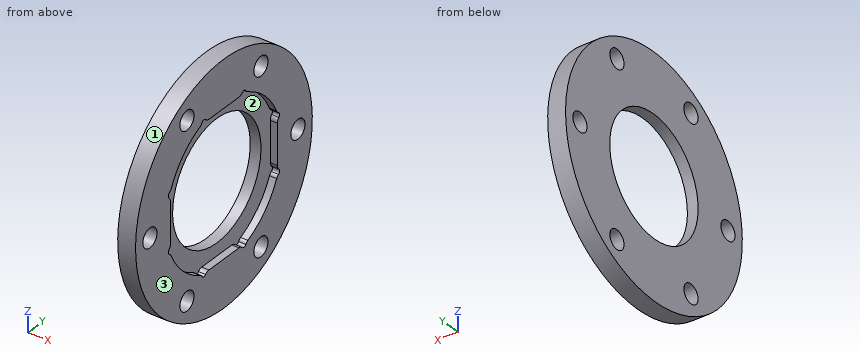
```python
from build123d import *

# Parameters (mm, degrees)
SKETCH_3_R          = 20
EXTRUDE_3_DEPTH     = 3
SKETCH_4_R          = 13.1
CUT_EXTRUDE_1_DEPTH = 1.2
EXTRUDE_START       = 1.2
EXTRUDE_4_DEPTH     = 1.2
SKETCH_6_R          = 10
CUT_EXTRUDE_2_DEPTH = 29.341489022
SKETCH_7_R          = 1.6
CUT_EXTRUDE_4_DEPTH = 29.442925307
SKETCH_8_R          = 0.5
CUT_EXTRUDE_5_DEPTH = 1.2
FILLET_START        = 1.8
FILLET_1_DEPTH      = 2.2


with BuildPart() as part:
    # 草图3 → 凸台-拉伸3 (new body)
    with BuildSketch(Plane(origin=(0, 0, 0), x_dir=(0, 0, -1), z_dir=(1, 0, 0))):
        Circle(SKETCH_3_R)
    extrude(amount=EXTRUDE_3_DEPTH)

    # 草图4 → 切除-拉伸1 (cut)
    with BuildSketch(Plane(origin=(3, 0, 0), x_dir=(0, 0, -1), z_dir=(1, 0, 0))):
        Circle(SKETCH_4_R)
    extrude(amount=-CUT_EXTRUDE_1_DEPTH, mode=Mode.SUBTRACT)

    # 草图5 → 凸台-拉伸4 (add)
    with BuildSketch(Plane(origin=(1.8, 0, 0), x_dir=(0, 0, -1), z_dir=(1, 0, 0)).offset(EXTRUDE_START)):
        with BuildLine():
            Line((-5.019960159, 12.1), (5.019960159, 12.1))
            ThreePointArc((5.019960159, 12.1), (0, 13.1), (-5.019960159, 12.1))
        make_face()
        with BuildLine():
            Line((-12.1, 5.019960159), (-12.1, -5.019960159))
            ThreePointArc((-12.1, -5.019960159), (-13.1, 0), (-12.1, 5.019960159))
        make_face()
        with BuildLine():
            Line((-5.019960159, -12.1), (5.019960159, -12.1))
            ThreePointArc((5.019960159, -12.1), (0, -13.1), (-5.019960159, -12.1))
        make_face()
        with BuildLine():
            Line((12.1, 5.019960159), (12.1, -5.019960159))
            ThreePointArc((12.1, -5.019960159), (13.1, 0), (12.1, 5.019960159))
        make_face()
    extrude(amount=-EXTRUDE_4_DEPTH)

    # 草图6 → 切除-拉伸2 (cut, through all)
    with BuildSketch(Plane(origin=(1.8, 0, 0), x_dir=(0, 0, -1), z_dir=(1, 0, 0))):
        Circle(SKETCH_6_R)
    extrude(amount=-CUT_EXTRUDE_2_DEPTH, mode=Mode.SUBTRACT)

    # 草图7 → 切除-拉伸4 (cut, through all)
    with BuildSketch(Plane(origin=(3, 0, 0), x_dir=(0, 0, -1), z_dir=(1, 0, 0))):
        with Locations((0, 16.75)):
            Circle(SKETCH_7_R)
        with Locations((14.505925513, 8.375)):
            Circle(SKETCH_7_R)
        with Locations((14.505925513, -8.375)):
            Circle(SKETCH_7_R)
        with Locations((0, -16.75)):
            Circle(SKETCH_7_R)
        with Locations((-14.505925513, -8.375)):
            Circle(SKETCH_7_R)
        with Locations((-14.505925513, 8.375)):
            Circle(SKETCH_7_R)
    extrude(amount=-CUT_EXTRUDE_4_DEPTH, mode=Mode.SUBTRACT)

    # 草图8 → 切除-拉伸5 (cut)
    with BuildSketch(Plane(origin=(3, 0, 0), x_dir=(0, 0, -1), z_dir=(1, 0, 0))):
        with Locations((-4.519960159, 12.1)):
            Circle(SKETCH_8_R)
        with Locations((12.1, 4.519960159)):
            Circle(SKETCH_8_R)
        with Locations((4.519960159, -12.1)):
            Circle(SKETCH_8_R)
        with Locations((-12.1, -4.519960159)):
            Circle(SKETCH_8_R)
        with Locations((4.519960159, 12.1)):
            Circle(SKETCH_8_R)
        with Locations((12.1, -4.519960159)):
            Circle(SKETCH_8_R)
        with Locations((-4.519960159, -12.1)):
            Circle(SKETCH_8_R)
        with Locations((-12.1, 4.519960159)):
            Circle(SKETCH_8_R)
    extrude(amount=-CUT_EXTRUDE_5_DEPTH, mode=Mode.SUBTRACT)

    # 圆角1: read off the stored shape, not the designer's step
    # 圆角1 outline → 圆角1 (cut)
    with BuildSketch(Plane.YZ.offset(FILLET_START)):
        with BuildLine():
            ThreePointArc((3.40192617, -12.1), (3.810174461, -12.187129071), (4.147282163, -12.433333333))
            ThreePointArc((4.147282163, -12.433333333), (4.05287398, -12.278411045), (4.019960159, -12.1))
            Line((4.019960159, -12.1), (3.40192617, -12.1))
        make_face()
        with BuildLine():
            ThreePointArc((5.019960159, -12.1), (5.003372821, -12.227719215), (4.954711368, -12.346964343))
            ThreePointArc((4.954711368, -12.346964343), (5.149921864, -12.102428131), (5.411148977, -11.930191396))
            ThreePointArc((5.411148977, -11.930191396), (5.216245603, -12.016687639), (5.019960159, -12.1))
        make_face()
        with BuildLine():
            ThreePointArc((-4.147282163, -12.433333333), (-3.810174461, -12.187129071), (-3.40192617, -12.1))
            Line((-3.40192617, -12.1), (-4.019960159, -12.1))
            ThreePointArc((-4.019960159, -12.1), (-4.05287398, -12.278411045), (-4.147282163, -12.433333333))
        make_face()
        with BuildLine():
            ThreePointArc((12.1, -5.019960159), (12.016687639, -5.216245603), (11.930191396, -5.411148977))
            ThreePointArc((11.930191396, -5.411148977), (12.102428131, -5.149921864), (12.346964343, -4.954711368))
            ThreePointArc((12.346964343, -4.954711368), (12.227719215, -5.003372821), (12.1, -5.019960159))
        make_face()
        with BuildLine():
            ThreePointArc((-5.411148977, -11.930191396), (-5.149921864, -12.102428131), (-4.954711368, -12.346964343))
            ThreePointArc((-4.954711368, -12.346964343), (-5.003372821, -12.227719215), (-5.019960159, -12.1))
            ThreePointArc((-5.019960159, -12.1), (-5.216245603, -12.016687639), (-5.411148977, -11.930191396))
        make_face()
        with BuildLine():
            ThreePointArc((12.1, -4.019960159), (12.278411045, -4.05287398), (12.433333333, -4.147282163))
            ThreePointArc((12.433333333, -4.147282163), (12.187129071, -3.810174461), (12.1, -3.40192617))
            Line((12.1, -3.40192617), (12.1, -4.019960159))
        make_face()
        with BuildLine():
            ThreePointArc((-12.346964343, -4.954711368), (-12.102428131, -5.149921864), (-11.930191396, -5.411148977))
            ThreePointArc((-11.930191396, -5.411148977), (-12.016687639, -5.216245603), (-12.1, -5.019960159))
            ThreePointArc((-12.1, -5.019960159), (-12.227719215, -5.003372821), (-12.346964343, -4.954711368))
        make_face()
        with BuildLine():
            Line((12.1, 4.019960159), (12.1, 3.40192617))
            ThreePointArc((12.1, 3.40192617), (12.187129071, 3.810174461), (12.433333333, 4.147282163))
            ThreePointArc((12.433333333, 4.147282163), (12.278411045, 4.05287398), (12.1, 4.019960159))
        make_face()
        with BuildLine():
            ThreePointArc((-12.1, -3.40192617), (-12.187129071, -3.810174461), (-12.433333333, -4.147282163))
            ThreePointArc((-12.433333333, -4.147282163), (-12.278411045, -4.05287398), (-12.1, -4.019960159))
            Line((-12.1, -4.019960159), (-12.1, -3.40192617))
        make_face()
        with BuildLine():
            ThreePointArc((12.1, 5.019960159), (12.227719215, 5.003372821), (12.346964343, 4.954711368))
            ThreePointArc((12.346964343, 4.954711368), (12.102428131, 5.149921864), (11.930191396, 5.411148977))
            ThreePointArc((11.930191396, 5.411148977), (12.016687639, 5.216245603), (12.1, 5.019960159))
        make_face()
        with BuildLine():
            ThreePointArc((-12.433333333, 4.147282163), (-12.187129071, 3.810174461), (-12.1, 3.40192617))
            Line((-12.1, 3.40192617), (-12.1, 4.019960159))
            ThreePointArc((-12.1, 4.019960159), (-12.278411045, 4.05287398), (-12.433333333, 4.147282163))
        make_face()
        with BuildLine():
            ThreePointArc((5.019960159, 12.1), (5.216245603, 12.016687639), (5.411148977, 11.930191396))
            ThreePointArc((5.411148977, 11.930191396), (5.149921864, 12.102428131), (4.954711368, 12.346964343))
            ThreePointArc((4.954711368, 12.346964343), (5.003372821, 12.227719215), (5.019960159, 12.1))
        make_face()
        with BuildLine():
            ThreePointArc((-11.930191396, 5.411148977), (-12.102428131, 5.149921864), (-12.346964343, 4.954711368))
            ThreePointArc((-12.346964343, 4.954711368), (-12.227719215, 5.003372821), (-12.1, 5.019960159))
            ThreePointArc((-12.1, 5.019960159), (-12.016687639, 5.216245603), (-11.930191396, 5.411148977))
        make_face()
        with BuildLine():
            ThreePointArc((4.019960159, 12.1), (4.05287398, 12.278411045), (4.147282163, 12.433333333))
            ThreePointArc((4.147282163, 12.433333333), (3.810174461, 12.187129071), (3.40192617, 12.1))
            Line((3.40192617, 12.1), (4.019960159, 12.1))
        make_face()
        with BuildLine():
            ThreePointArc((-4.954711368, 12.346964343), (-5.149921864, 12.102428131), (-5.411148977, 11.930191396))
            ThreePointArc((-5.411148977, 11.930191396), (-5.216245603, 12.016687639), (-5.019960159, 12.1))
            ThreePointArc((-5.019960159, 12.1), (-5.003372821, 12.227719215), (-4.954711368, 12.346964343))
        make_face()
        with BuildLine():
            Line((-4.019960159, 12.1), (-3.40192617, 12.1))
            ThreePointArc((-3.40192617, 12.1), (-3.810174461, 12.187129071), (-4.147282163, 12.433333333))
            ThreePointArc((-4.147282163, 12.433333333), (-4.05287398, 12.278411045), (-4.019960159, 12.1))
        make_face()
    extrude(amount=FILLET_1_DEPTH, mode=Mode.SUBTRACT)


solid = part.part
```
Source: CAD feature listing. Evaluate the final solid. Frame: model axes, mm. Face numbers are marked on the shaded views. Coordinates: 2 decimals unless noted, no trailing zeros. Loops run counter-clockwise (first coordinate to the right, second up) from the corner with the lowest first, then second, coordinate; pieces in that order, holes last. Notation, with made-up numbers: (51.25, -27) - (58.25, -27) arc R23 ccw to (58.25, 11) - close; hole circle Ø4 at (-34.75, 26). An arc over 180 degrees is marked (long way). Answer as CSV lines item,"result".
1. Section B-B (z = 0). Return loops of the section in (x, y).
Established:
outline,"(0, -20) - (3, -20) - (3, -18.35) - (0, -18.35) - close; (0, -15.15) - (3, -15.15) - (3, -12.1) - (1.8, -12.1) - (1.8, -10) - (0, -10) - close; (0, 10) - (1.8, 10) - (1.8, 12.1) - (3, 12.1) - (3, 15.15) - (0, 15.15) - close; (0, 18.35) - (3, 18.35) - (3, 20) - (0, 20) - close"
2. Mould query, pull axis Z, two halves, no side actions, for the marked faces 1, 2 and 3. Classes: released by +Z, released by -Z, zero draft, split by the parting line, or undercut.
Established:
face 1,"split by the parting line"
face 2,"undercut"
face 3,"zero draft"
3. Contact query for flat-ended pins moving along their axis: pin 1 (1.9 mm diameter, centred on y = 8.38, z = -14.51, fed in from -X); pin 2 (12 mm diameter, centred on y = 4, z = 1.5, fed in from +X); pin 3 (0.6 mm diameter, centred on x = 2, z = -1, fed in from +Y); pin 4 (1 mm diameter, centred on x = 2.5, z = -1, fed in from -Y). Output: stop coordinate, or through.
Established:
pin 1,"passes through"
pin 2,"stops at x = 1.8"
pin 3,"stops at y = 19.99"
pin 4,"stops at y = -19.99"
4. Section A-A (y = 0). Return loops of the section in (x, z).
Established:
outline,"(0, -20) - (3, -20) - (3, -12.1) - (1.8, -12.1) - (1.8, -10) - (0, -10) - close; (0, 10) - (1.8, 10) - (1.8, 12.1) - (3, 12.1) - (3, 20) - (0, 20) - close"
5. Section C-C (x = 0.8). Return loops of the section in (y, z) (3 decimals), then the cut area to 3 significant figures.
Established:
outline,"circle Ø40 at (0, 0); hole circle Ø3.2 at (-16.75, 0); hole circle Ø20 at (0, 0); hole circle Ø3.2 at (-8.375, -14.506); hole circle Ø3.2 at (-8.375, 14.506); hole circle Ø3.2 at (8.375, -14.506); hole circle Ø3.2 at (8.375, 14.506); hole circle Ø3.2 at (16.75, 0)"
area,"894 mm2"
6. Section D-D (z = -6.5). Return loops of the section in (x, y), then the cut area to 3 significant figures.
Established:
outline,"(0, -18.91) - (3, -18.91) - (3, -11.37) - (1.8, -11.37) - (1.8, -7.6) - (0, -7.6) - close; (0, 7.6) - (1.8, 7.6) - (1.8, 11.37) - (3, 11.37) - (3, 18.91) - (0, 18.91) - close"
area,"58.8 mm2"
7. Ray query, line 1 (Y direction, x = 0.5, z = 0); line 2 (Z direction, x = 2.5, y = 7) (3 decimals); line 3 (Y direction, x = 2.35, z = -13.5). Return the intervals inside material, ascending.
Established:
line 1,"y = -20 to -18.35, -15.15 to -10, 10 to 15.15, 18.35 to 20"
line 2,"z = -18.735 to -15.324, -13.688 to -11.073, 11.073 to 13.688, 15.324 to 18.735"
line 3,"y = -14.76 to -9.62, -7.13 to 7.13, 9.62 to 14.76"
